Can you work these out from the drawing? Everything is in mm from the part's minimum corner. Round coordinates to 2 decimals unless told otherwise and drop trailing zeros. Order: outer loops, then holes, each group sorted by start corner. A loop starts at its lowest first (then second) coordinate and runs counter-clockwise, first axis right, second up. Notation, with made-up numbers: (-19, -22.5) -> (5, -22.5) arc R19 ccw to (5, -8.5) -> close; hole circle Ø7 at (38.25, 0.25). An arc over 180 degrees is marked (long way). One line per item, written item: value.
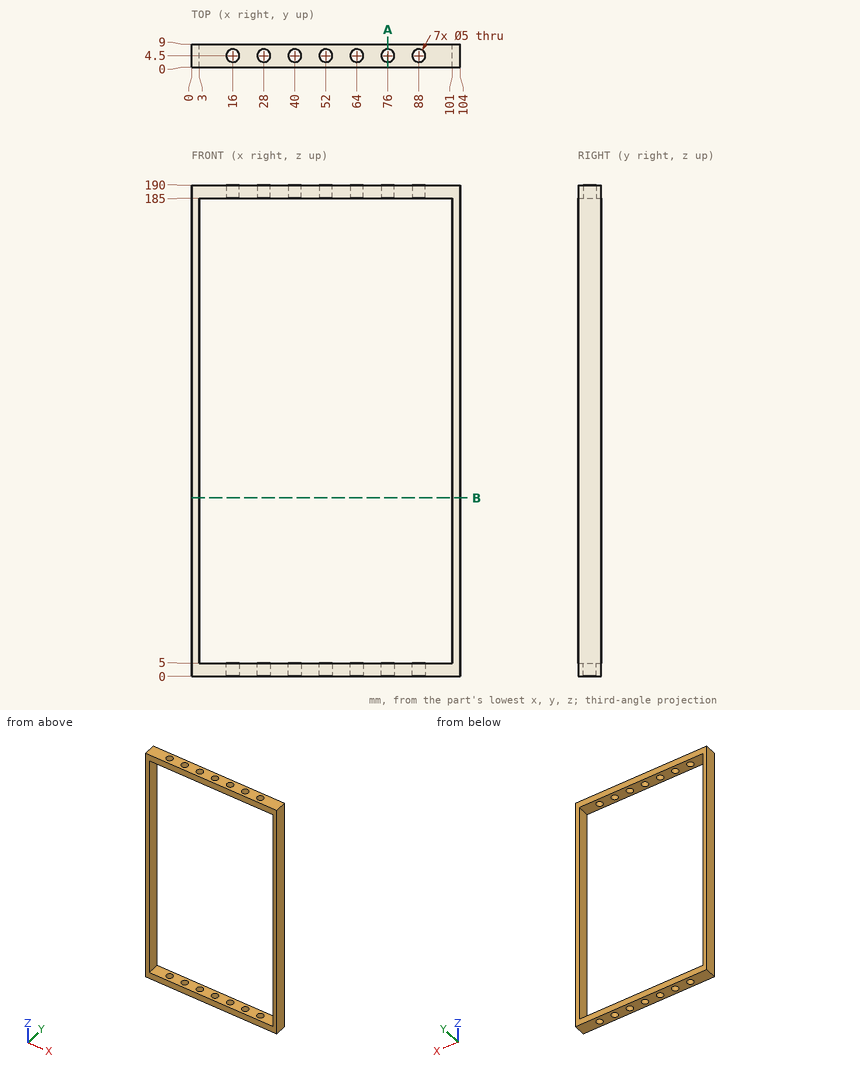
Q1. Will these pins go through, and if not, where does the flat tip stop? pin 1 Ø4 at (x, y) = (52, 4.5) entering from -Z; pin 2 Ø1 at (x, y) = (30.5, 7.5) entering from -Z.
Answers below:
pin 1: through
pin 2: z = 0
Q2. I want a section at A-A on x = 76. List the corners of the cut face in (y, z) for me, plus the area to 3 significant figures.
Answers below:
outline: (0, 0) -> (2, 0) -> (2, 5) -> (0, 5) -> close; (0, 185) -> (2, 185) -> (2, 190) -> (0, 190) -> close; (7, 0) -> (9, 0) -> (9, 5) -> (7, 5) -> close; (7, 185) -> (9, 185) -> (9, 190) -> (7, 190) -> close
area: 40.0 mm^2
Q3. Please list where these lines run through material, in increasing order: line 1 along Z through (x, y) = (98.5, 6); line 2 along X through (y, z) = (1.75, 71); line 3 along Y through (x, z) = (88, 186.1).
Answers below:
line 1: 0 to 5, 185 to 190
line 2: 0 to 3, 101 to 104
line 3: 0 to 2, 7 to 9
Q4. I want a section at B-B on z = 69. List the corners of the cut face in (x, y) for me.
Answers below:
outline: (0, 0) -> (3, 0) -> (3, 9) -> (0, 9) -> close; (101, 0) -> (104, 0) -> (104, 9) -> (101, 9) -> close
